from build123d import *

# Parameters (mm, degrees)
F0_W      = 247.65
F0_H      = 304.8
F1_DEPTH  = 12.7
F2_W      = 2.54
F2_H      = 63.5
F3_DEPTH  = 152.4
F4_W      = 76.2
F4_H      = 2.54
F5_DEPTH  = 152.4
F6_W      = 42.164
F6_H      = 63.5
F7_DEPTH  = 76.2
F8_W      = 33.782
F8_H      = 63.5
F9_DEPTH  = 63.5
F10_W     = 5.08
F10_H     = 88.9
F11_DEPTH = 63.5
F12_W     = 31.75
F12_H     = 76.2
F13_DEPTH = 127
F14_W     = 31.75
F14_H     = 42.164
F15_DEPTH = 38.1
F16_W     = 127
F16_H     = 165.1
F17_DEPTH = 50.8


with BuildPart() as f1:
    # F0 (on Top) → F1 (new body)
    with BuildSketch(Plane.XY):
        with Locations((123.825, -152.4)):
            Rectangle(F0_W, F0_H)
    extrude(amount=F1_DEPTH)

    # F2 (on face) → F3 (join)
    with BuildSketch(Plane.XY.offset(12.7)):
        with Locations((1.27, -76.2)):
            Rectangle(F2_W, F2_H)
    extrude(amount=F3_DEPTH)

    # F4 (on face) → F5 (join)
    with BuildSketch(Plane.XY.offset(12.7)):
        with Locations((76.2, -1.27)):
            Rectangle(F4_W, F4_H)
    extrude(amount=F5_DEPTH)

    # F6 (on face) → F7 (join)
    with BuildSketch(Plane.XY.offset(12.7)):
        Polygon((247.65, -42.164), (247.65, 0), (146.05, 0), (146.05, -42.164), (205.486, -42.164), align=None)
        with Locations((226.568, -73.914)):
            Rectangle(F6_W, F6_H)
    extrude(amount=F7_DEPTH)

    # F8 (on face) → F9 (join)
    with BuildSketch(Plane.XY.offset(12.7)):
        with Locations((230.759, -146.05)):
            Rectangle(F8_W, F8_H)
    extrude(amount=F9_DEPTH)

    # F10 (on face) → F11 (join)
    with BuildSketch(Plane.XY.offset(76.2)):
        with Locations((226.06, -152.4)):
            Rectangle(F10_W, F10_H)
    extrude(amount=F11_DEPTH)

    # F12 (on face) → F13 (join)
    with BuildSketch(Plane.XY.offset(12.7)):
        with Locations((231.775, -266.7)):
            Rectangle(F12_W, F12_H)
    extrude(amount=F13_DEPTH)

    # F14 (on face) → F15 (join)
    with BuildSketch(Plane.XY.offset(12.7)):
        with Locations((225.425, -207.518)):
            Rectangle(F14_W, F14_H)
    extrude(amount=F15_DEPTH)

    # F16 (on face) → F17 (join)
    with BuildSketch(Plane.XY.offset(12.7)):
        with Locations((63.5, -222.25)):
            Rectangle(F16_W, F16_H)
    extrude(amount=F17_DEPTH)


solid = f1.part
Verification items for the finished model (mm, model axes). A direction names the side the tool comes from. Coordinates: 2 decimals unless noted, no trailing zeros. Order: outer loops, then holes, each group sorted by start corner. A loop starts at its lowest first (then second) coordinate and runs counter-clockwise, first axis right, second up.
Item 1: Section check C-C, the plane z = 146. Enter the section's corners in (x, y).
Filled in:
outline: (0, -107.95) - (2.54, -107.95) - (2.54, -44.45) - (0, -44.45) - close; (38.1, -2.54) - (114.3, -2.54) - (114.3, 0) - (38.1, 0) - close
Item 2: Depth check by flat-ended pin: pin 1 (9.5 mm diameter, centred on x = 233, y = -272, fed in from +Z); pin 2 (9.5 mm diameter, centred on x = 237, y = -140.5, fed in from +Z); pin 3 (21 mm diameter, centred on y = -23, z = 56, fed in from -X). Enter the tip coordinate at first touch or a pass-through.
Filled in:
pin 1: stops at z = 139.7
pin 2: stops at z = 76.2
pin 3: stops at x = 146.05
Item 3: Release check for a two-part mould opening along X. For faces 4 (the face through (175, -42.164, 50)), 5 (the face through (215.9, -267, 75)), 6 (the face through (247.65, -155, 53)), 7 (the face through (223.52, -153, 108)) record: +X half, -X half, draft (parallel to the pull), parting line (faces both ways), or undercut.
Filled in:
face 4: draft
face 5: undercut
face 6: +X half
face 7: -X half
Item 4: Section check D-D, the plane y = -85. Enter the section's corners in (x, z), then the cut area to 3 significant figures.
Filled in:
outline: (0, 0) - (247.65, 0) - (247.65, 88.9) - (205.49, 88.9) - (205.49, 12.7) - (2.54, 12.7) - (2.54, 165.1) - (0, 165.1) - close
area: 6,750 mm2
Item 5: Section check A-A, the plane y = -182. Enter the section's corners in (x, z).
Filled in:
outline: (0, 0) - (247.65, 0) - (247.65, 12.7) - (127, 12.7) - (127, 63.5) - (0, 63.5) - close; (223.52, 76.2) - (228.6, 76.2) - (228.6, 139.7) - (223.52, 139.7) - close
Item 6: Material ranges on L1, parallel to X at y = -211, z = 35; L2, parallel to X at y = -99.5, z = 42; L3, parallel to Y at x = 74.5, z = 23.5, recorded low to high.
Filled in:
L1: x = 0 to 127, 209.55 to 241.3
L2: x = 0 to 2.54, 205.49 to 247.65
L3: y = -304.8 to -139.7, -2.54 to 0
Item 7: Section check B-B, the plane z = 121. Enter the section's corners in (x, y), then the cut area to 3 significant figures.
Filled in:
outline: (0, -107.95) - (2.54, -107.95) - (2.54, -44.45) - (0, -44.45) - close; (38.1, -2.54) - (114.3, -2.54) - (114.3, 0) - (38.1, 0) - close; (215.9, -304.8) - (247.65, -304.8) - (247.65, -228.6) - (215.9, -228.6) - close; (223.52, -196.85) - (228.6, -196.85) - (228.6, -107.95) - (223.52, -107.95) - close
area: 3,230 mm2
Item 8: Access from +Z, -Z, +X, -X, +Y, -Y to the whole of each face (thin tool, end or side, straight path). Record for faces 1 (the face through (2.54, -77, 88)), 2 (the face through (209.55, -208, 31)), 3 (the face through (76, -2.54, 88)).
Filled in:
face 1: +Z, +Y
face 2: +Z, -Y
face 3: +Z, -X
